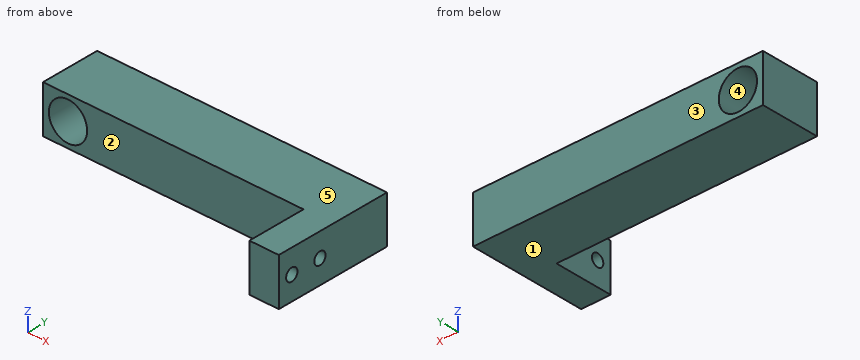
```python
from build123d import *

# Parameters (mm, degrees)
SKETCH_1_W          = 88.5
SKETCH_1_H          = 16
SKETCH_1_R          = 6.5
EXTRUDE_1_DEPTH     = 20
SKETCH_2_W          = 16
SKETCH_2_H          = 40
EXTRUDE_2_DEPTH     = 10
SKETCH_3_R          = 2.1
CUT_EXTRUDE_1_DEPTH = 10


with BuildPart() as part:
    # 草图1 → 凸台-拉伸1 (new body)
    with BuildSketch(Plane(origin=(0, 0, 0), x_dir=(1, 0, 0), z_dir=(0, 1, 0))):
        with Locations((35.75, 0)):
            Rectangle(SKETCH_1_W, SKETCH_1_H)
        Circle(SKETCH_1_R, mode=Mode.SUBTRACT)
    extrude(amount=EXTRUDE_1_DEPTH)

    # 草图2 → 凸台-拉伸2 (add)
    with BuildSketch(Plane(origin=(80, 0, 0), x_dir=(0, 0, -1), z_dir=(1, 0, 0))):
        Rectangle(SKETCH_2_W, SKETCH_2_H)
    extrude(amount=EXTRUDE_2_DEPTH)

    # 草图3 → 切除-拉伸1 (cut)
    with BuildSketch(Plane.ZY.offset(-80)):
        with Locations((0, -4.8)):
            Circle(SKETCH_3_R)
        with Locations((0, -15.2)):
            Circle(SKETCH_3_R)
    extrude(amount=-CUT_EXTRUDE_1_DEPTH, mode=Mode.SUBTRACT)


solid = part.part
```
Read the model definition and answer for the solid it produces. Units are mm, in the model's axes. Face numbers are marked on the shaded views. A direction names the side the tool comes from. Coordinates: 2 decimals unless noted, no trailing zeros. Write each loop counter-clockwise with the first axis right and the second up, starting at its lowest first coordinate (ties: lowest second). Pieces come first, ordered by that corner, then holes. Notation, with made-up numbers: (39.25, -37) -> (66.25, -37) arc R18 cw to (66.25, -31) -> close; hole circle Ø11 at (10.5, -28). An arc over 180 degrees is marked (long way). Write item = value, one per line.
(1) Section B-B on x = 0 is taken. Write down the section's boundary in (y, z).
From the geometry:
outline = (0, -8) -> (20, -8) -> (20, -6.5) -> (0, -6.5) -> close; (0, 6.5) -> (20, 6.5) -> (20, 8) -> (0, 8) -> close
(2) Given pin 1 Ø8 at (y, z) = (-10.5, -3.5) entering from -X; pin 2 Ø8 at (x, z) = (0, 0) entering from +Y; pin 3 Ø5 at (x, z) = (49.5, -1) entering from -Y, each flat-ended and moving along its own axis, determine where each tip first touches the part or whether it passes through.
From the geometry:
pin_1 = 80
pin_2 = through
pin_3 = 0
(3) Straight lines are drawn through the part: L1, parallel to Y at x = 83.25, z = 0; L2, parallel to Z at x = 0, y = 12; L3, parallel to X at y = 11, z = 0. For each, find the intervals that lie inside material, in ascending order. Write a range as from..to.
From the geometry:
L1 = -20..-17.3, -13.1..-6.9, -2.7..20
L2 = -8..-6.5, 6.5..8
L3 = -8.5..-6.5, 6.5..90
(4) Section A-A on z = 0 is taken. Write down the section's boundary in (x, y).
From the geometry:
outline = (-8.5, 0) -> (-6.5, 0) -> (-6.5, 20) -> (-8.5, 20) -> close; (6.5, 0) -> (80, 0) -> (80, -2.7) -> (90, -2.7) -> (90, 20) -> (6.5, 20) -> close; (80, -20) -> (90, -20) -> (90, -17.3) -> (80, -17.3) -> close; (80, -13.1) -> (90, -13.1) -> (90, -6.9) -> (80, -6.9) -> close
(5) Section C-C on y = -4.8 is taken. Write down the section's boundary in (x, z), plus the area to 3 significant figures.
From the geometry:
outline = (80, -8) -> (90, -8) -> (90, -2.1) -> (80, -2.1) -> close; (80, 2.1) -> (90, 2.1) -> (90, 8) -> (80, 8) -> close
area = 118 mm2
(6) For a pull along Z with two mould halves and no side action, classify the marked faces 3, 4 and 5 as +Z half, -Z half, draft (parallel to the pull), parting line (faces both ways), or undercut.
From the geometry:
face_3 = draft
face_4 = undercut
face_5 = +Z half
(7) Section D-D on y = 15 is taken. Write down the section's boundary in (x, z).
From the geometry:
outline = (-8.5, -8) -> (90, -8) -> (90, 8) -> (-8.5, 8) -> close; hole circle Ø13 at (0, 0)
(8) Which of the six approach directions +Z, -Z, +X, -X, +Y, -Y give full straight-line access (tool end or side, diameter ignored) to the marked faces 1 and 2?
From the geometry:
face_1 = -Z, +X, -X, +Y, -Y
face_2 = +Z, -Z, -X, -Y
